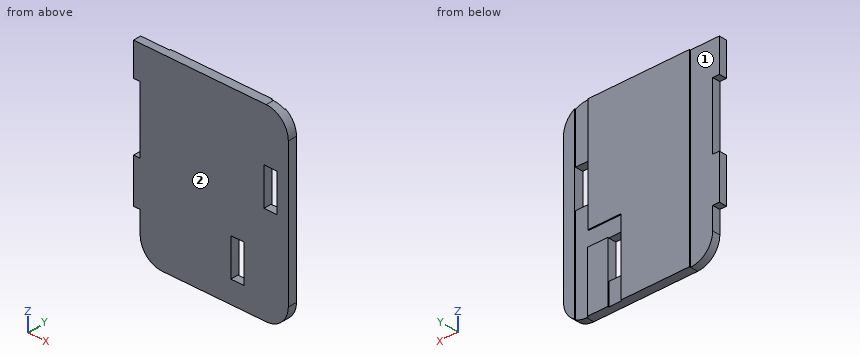
```python
from build123d import *

# Parameters (mm, degrees)
SKETCH1_W           = 0.6
SKETCH1_H           = 1.7
BOSS_EXTRUDE1_DEPTH = 0.4
FILLET2_R           = 1
SKETCH2_W           = 1.780104135
SKETCH2_H           = 8.5
CUT_EXTRUDE1_DEPTH  = 0.05


with BuildPart() as part:
    # Sketch1 → Boss-Extrude1 (new body)
    with BuildSketch(Plane(origin=(0, 0, 0), x_dir=(1, 0, 0), z_dir=(0, 1, 0))):
        Polygon((0, 0), (7, 0), (7, 8.5), (0.3, 8.5), (0.3, 6.5), (0, 6.5), (0, 4.5), (0.3, 4.5), (0.3, 1.5), (0, 1.5), align=None)
        with Locations((4.7, 6.65)):
            Rectangle(SKETCH1_W, SKETCH1_H, mode=Mode.SUBTRACT)
        with Locations((6.2, 3.25)):
            Rectangle(SKETCH1_W, SKETCH1_H, mode=Mode.SUBTRACT)
    extrude(amount=BOSS_EXTRUDE1_DEPTH)

    # Fillet2
    fillet2_edges = [part.edges().sort_by_distance(p)[0] for p in [
        (0.3, 0.2, -8.5),
        (7, 0.2, -8.5),
        (7, 0.2, 0),
    ]]
    fillet(fillet2_edges, radius=FILLET2_R)

    # Sketch2 → Cut-Extrude1 (cut)
    with BuildSketch(Plane(origin=(0, 0.4, 0), x_dir=(1, 0, 0), z_dir=(0, 1, 0))):
        with Locations((0.409947933, 4.25)):
            Rectangle(SKETCH2_W, SKETCH2_H)
        Polygon((4.4, 7.5), (4.4, 8.794208179), (5, 8.794208179), (5, 7.5), (5, 5.8), (5.909455283, 5.8), (5.909455283, 8.5), (6.5, 8.5), (6.5, 5.123047138), (6.5, 4.1), (6.5, 0), (5.9, 0), (5.9, 4.1), (5.9, 5.123047138), (4.4, 5.123047138), align=None)
    extrude(amount=-CUT_EXTRUDE1_DEPTH, mode=Mode.SUBTRACT)


solid = part.part
```
Here's how the part is built. I have some questions about the finished solid (model axes, mm). Face numbers are marked on the shaded views. A direction names the side the tool comes from. Coordinates: 2 decimals unless noted, no trailing zeros. Loops run counter-clockwise (first coordinate to the right, second up) from the corner with the lowest first, then second, coordinate; pieces in that order, holes last. Notation, with made-up numbers: (63, -27.5) - (98, -27.5) arc R20 ccw to (98, -22.5) - close; hole circle Ø9 at (37, -22). An arc over 180 degrees is marked (long way). Return JSON: item names as keys, results as strings. Group by question number.
Item 1: On a 3-axis mill with a long thin cutter (end or side, diameter ignored), from which of +Z, -Z, +X, -X, +Y, -Y can I reach the whole of each face in a straight line? I mean the marked faces 1 and 2. Say none if no direction works.
Item 2: I need wall thicknesses on line 1 (X direction, y = 0.25, z = -7); line 2 (X direction, y = 0.2, z = -4); line 3 (Z direction, x = 4.75, y = 0.15). Which ranges of each line are inside material? Lowest first, please. Write a range as from..to.
Item 3: If we section it at D-D on z = -4.25: Write out the boundary of the cut face in (x, y).
Item 4: If we section it at C-C on y = 0.1: Write out the boundary of the cut face in (x, z).
Item 5: If we section it at A-A on x = 4.5: Write out the boundary of the cut face in (y, z), and give its area (3 significant figures).
Item 6: If we section it at B-B on z = -2.5: Write out the boundary of the cut face in (x, y), and give its area (3 significant figures).
Calculated:
{
 "1": {"face 1": "+Z, -Z, -X, +Y", "face 2": "+Z, -Z, +X, -X, -Y"},
 "2": {"line 1": "x = 0.3..4.4, 5..7", "line 2": "x = 0.3..5.9, 6.5..7", "line 3": "z = -8.5..-7.5, -5.8..0"},
 "3": {"outline": "(0.3, 0) - (7, 0) - (7, 0.4) - (6.5, 0.4) - (6.5, 0.35) - (5.9, 0.35) - (5.9, 0.4) - (1.3, 0.4) - (1.3, 0.35) - (0.3, 0.35) - close"},
 "4": {"outline": "(0, -6.5) - (0.3, -6.5) - (0.3, -7.5) arc R1 ccw to (1.3, -8.5) - (6, -8.5) arc R1 ccw to (7, -7.5) - (7, -1) arc R1 ccw to (6, 0) - (0, 0) - (0, -1.5) - (0.3, -1.5) - (0.3, -4.5) - (0, -4.5) - close; hole (4.4, -7.5) - (5, -7.5) - (5, -5.8) - (4.4, -5.8) - close; hole (5.9, -4.1) - (6.5, -4.1) - (6.5, -2.4) - (5.9, -2.4) - close"},
 "5": {"outline": "(0, -8.5) - (0.35, -8.5) - (0.35, -7.5) - (0, -7.5) - close; (0, -5.8) - (0.35, -5.8) - (0.35, -5.12) - (0.4, -5.12) - (0.4, 0) - (0, 0) - close", "area": "2.64 mm^2"},
 "6": {"outline": "(0.3, 0) - (5.9, 0) - (5.9, 0.4) - (1.3, 0.4) - (1.3, 0.35) - (0.3, 0.35) - close; (6.5, 0) - (7, 0) - (7, 0.4) - (6.5, 0.4) - close", "area": "2.39 mm^2"}
}
